from build123d import *

# Parameters (mm, degrees)
ESQUISSE2_OUTSIDE_W     = 34.974
ESQUISSE2_OUTSIDE_H     = 34.974
ENL_V_MAT_EXTRU_1_DEPTH = 10.8
CHANFREIN_SIZE          = 1.75


with BuildPart() as part:
    # Esquisse1 → Base-R_volution (revolve)
    with BuildSketch(Plane.XY, mode=Mode.PRIVATE) as base_r_volution_sk:
        Polygon((4.484455543, 10.8), (9, 10.8), (12.727922061, 8.647683156), (12.727922061, 2.152316844), (9, 0), (4.484455543, 0), align=None)
    revolve(base_r_volution_sk.sketch.rotate(Axis((0, 2.4, 0), (0, -1, 0)), 90), axis=Axis((0, 2.4, 0), (0, -1, 0)))

    # Esquisse2 outside → Enl_v. mat.-Extru.1 (cut)
    with BuildSketch(Plane(origin=(0, 0, 0), x_dir=(1, 0, 0), z_dir=(0, 1, 0))):
        Rectangle(ESQUISSE2_OUTSIDE_W, ESQUISSE2_OUTSIDE_H)
        Polygon((-5.196152423, -9), (5.196152423, -9), (10.392304845, 0), (5.196152423, 9), (-5.196152423, 9), (-10.392304845, 0), align=None, mode=Mode.SUBTRACT)
    extrude(amount=ENL_V_MAT_EXTRU_1_DEPTH, mode=Mode.SUBTRACT)

    # Chanfrein
    chanfrein_edges = [part.edges().sort_by_distance(p)[0] for p in [
        (0, 10.8, -4.484455543),
        (0, 0, -4.484455543),
    ]]
    chamfer(chanfrein_edges, length=CHANFREIN_SIZE)


solid = part.part
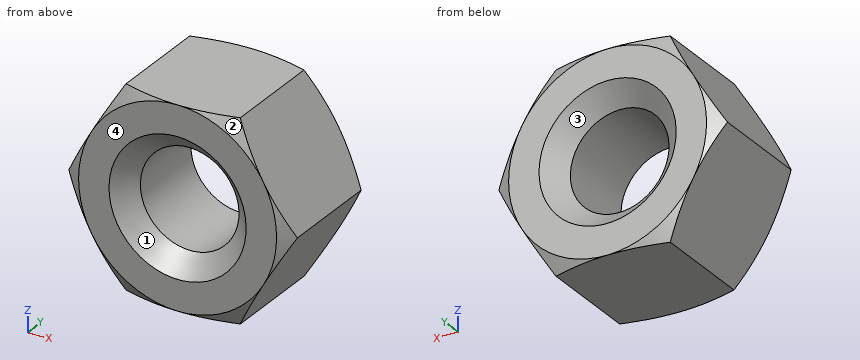
Here's how the part is built. I have some questions about the finished solid (model axes, mm). Face numbers are marked on the shaded views. Round coordinates to 2 decimals unless told otherwise and drop trailing zeros. Write each loop counter-clockwise with the first axis right and the second up, starting at its lowest first coordinate (ties: lowest second). Pieces come first, ordered by that corner, then holes.
1. If we mould it in two halves opening along Z, with no side actions, what happens to the marked faces 1, 2, 3 and 4? For each: released by +Z, released by -Z, zero draft, split by the parting line, or undercut.
2. Suppose I cut it at A-A (y = 6.75). List the corners of the cut face in (x, z) for me.
3. I need wall thicknesses on L1, parallel to X at y = 2.25, z = -3; L2, parallel to Z at x = -3.75, y = 9.5; L3, parallel to Z at x = -2.75, y = 6.25. Which ranges of each line are inside material? Lowest first, please.
4. Will these pins go through, and if not, where does the flat tip stop? pin 1 Ø4 at (y, z) = (2.5, -3.5) entering from +X; pin 2 Ø6 at (y, z) = (9.5, 4.5) entering from -X; pin 3 Ø4 at (x, y) = (-7.5, 6) entering from -Z; pin 4 Ø3 at (x, z) = (-5, 4) entering from -Y.
Answer sheet:
1. face 1: undercut
1. face 2: released by +Z
1. face 3: undercut
1. face 4: zero draft
2. outline: (-10.39, 0) - (-5.2, -9) - (5.2, -9) - (10.39, 0) - (5.2, 9) - (-5.2, 9) - close; hole circle Ø8.97 at (0, 0)
3. L1: x = -8.66 to -3.33, 3.33 to 8.66
3. L2: z = -9 to -3.21, 3.21 to 9
3. L3: z = -9 to -3.54, 3.54 to 9
4. pin 1: stops at x = 9.53
4. pin 2: stops at x = -9.53
4. pin 3: stops at z = -8.47
4. pin 4: stops at y = 0
